```python
from build123d import *

# Parameters (mm, degrees)
RACK_DEPTH             = 112.7125
RACK_DEPTH_BACK        = 112.7125
SKETCH2_R              = 4.7625
END_HOLE_DEPTH         = 25.4
BUMP_START             = -17.018
SKETCH3_R              = 11.3157
SKETCH3_R_2            = 10.31875
BUMP_STOP_DEPTH        = 0.9652
SKETCH4_R              = 0.762
SAFETY_WIRE_HOLE_DEPTH = 12.3157


with BuildPart() as part:
    # Sketch1 → Rack (new body, two sides)
    with BuildSketch(Plane.XY) as rack_sk:
        with BuildLine():
            Line((7.127857322, 7.46125), (-7.127857322, 7.46125))
            ThreePointArc((-7.127857322, 7.46125), (-4.057463729, -9.487549191), (10.31875, 0))
            ThreePointArc((10.31875, 0), (9.487549191, 4.057463729), (7.127857322, 7.46125))
        make_face()
    extrude(amount=RACK_DEPTH)
    extrude(rack_sk.sketch, amount=-RACK_DEPTH_BACK)

    # Sketch2 → End Hole (cut)
    with BuildSketch(Plane.XY.offset(112.7125)):
        Circle(SKETCH2_R)
    end_hole = extrude(amount=-END_HOLE_DEPTH, mode=Mode.SUBTRACT)

    # Sketch3 → Bump Stop (add)
    with BuildSketch(Plane.XY.offset(112.7125).offset(BUMP_START)):
        Circle(SKETCH3_R)
        Circle(SKETCH3_R_2, mode=Mode.SUBTRACT)
    bump_stop = extrude(amount=BUMP_STOP_DEPTH)

    # Sketch4 → Safety Wire Hole (cut, symmetric)
    with BuildSketch(Plane(origin=(0, 0, 0), x_dir=(0, 0, -1), z_dir=(1, 0, 0))):
        with Locations((-106.3625, 0)):
            Circle(SKETCH4_R)
    safety_wire_hole = extrude(amount=SAFETY_WIRE_HOLE_DEPTH, both=True, mode=Mode.SUBTRACT)

    # Rack Mirror: End Hole, Bump Stop, Safety Wire Hole across plane
    add(end_hole.mirror(Plane.XY), mode=Mode.SUBTRACT)
    add(bump_stop.mirror(Plane.XY))
    add(safety_wire_hole.mirror(Plane.XY), mode=Mode.SUBTRACT)


solid = part.part
```
Verification items for the finished model (mm, model axes). A direction names the side the tool comes from. Coordinates: 2 decimals unless noted, no trailing zeros. Write each loop counter-clockwise with the first axis right and the second up, starting at its lowest first coordinate (ties: lowest second). Pieces come first, ordered by that corner, then holes. Notation, with made-up numbers: (-35.75, 89.25) - (-0.75, 89.25) arc R23 cw to (-0.75, 119.25) - close; hole circle Ø10 at (3.5, 68). An arc over 180 degrees is marked (long way). One line per question, with ' | ' between items. Start each with the question number.
1. Gauge pin test, flat ends, axial feed: P1, Ø12.5, axis at x = 0, y = 0, coming from the +Z side; P2, Ø12, axis at x = -3.5, z = 72.5, coming from the +Y side; P3, Ø5, axis at x = -4.5, z = 86, coming from the -Y side; P4, Ø12, axis at x = -6.5, z = 52, coming from the -Y side. Record the tip position at first contact, or that the pin passes through.
2. Material ranges on line 1 along Z through (x, y) = (-8.9, 0); line 2 along Y through (x, z) = (0, -95.75); line 3 along Z through (x, y) = (-4, -10.5), recorded low to high.
3. Section check C-C (z = -68.5). Enter the section's corners in (x, y), plus the area to 3 significant figures.
4. Section check A-A (x = 0). Enter the section's corners in (y, z).
5. Access from +Z, -Z, +X, -X, +Y, -Y to the whole of each face (thin tool, end or side, straight path). Record for faces 4 (the cylindrical face through (-0.344, -10.313, 1.34)), 5 (the flat face through (5, -9.2, 96.66)), 6 (the cylindrical face through (-0.344, -10.313, -104.574)).
6. Draft check along Z on faces 1 (the cylindrical face through (10.793, 3.399, 96.17)), 2 (the flat face through (0, 0, -87.312)), 3 (the flat face through (5, -9.2, 95.694)). Enter one of: released by +Z, released by -Z, zero draft, split by the parting line, or undercut.
7. Section check B-B (z = 92). Enter the section's corners in (x, y) (1 decimal), plus the area to 3 significant figures.
Computed values:
1) P1: z = 112.71 | P2: y = 7.46 | P3: y = -10.12 | P4: y = -10.31
2) line 1: -112.71 to -107.12, -105.6 to 105.6, 107.12 to 112.71 | line 2: -11.32 to -4.76, 4.76 to 7.46, 10.32 to 11.32 | line 3: -96.66 to -95.69, 95.69 to 96.66
3) outline: (-7.13, 7.46) arc R10.32 ccw (long way) to (7.13, 7.46) - close | area: 306 mm²
4) outline: (-11.32, -96.66) - (-10.32, -96.66) - (-10.32, -112.71) - (-4.76, -112.71) - (-4.76, -87.31) - (4.76, -87.31) - (4.76, -112.71) - (7.46, -112.71) - (7.46, 112.71) - (4.76, 112.71) - (4.76, 87.31) - (-4.76, 87.31) - (-4.76, 112.71) - (-10.32, 112.71) - (-10.32, 96.66) - (-11.32, 96.66) - (-11.32, 95.69) - (-10.32, 95.69) - (-10.32, -95.69) - (-11.32, -95.69) - close; (10.32, -96.66) - (11.32, -96.66) - (11.32, -95.69) - (10.32, -95.69) - close; (10.32, 95.69) - (11.32, 95.69) - (11.32, 96.66) - (10.32, 96.66) - close
5) face 4: none | face 5: +Z | face 6: -Z
6) face 1: zero draft | face 2: released by -Z | face 3: undercut
7) outline: (-7.1, 7.5) arc R10.3 ccw (long way) to (7.1, 7.5) - close; hole circle Ø9.5 at (0, 0) | area: 235 mm²
